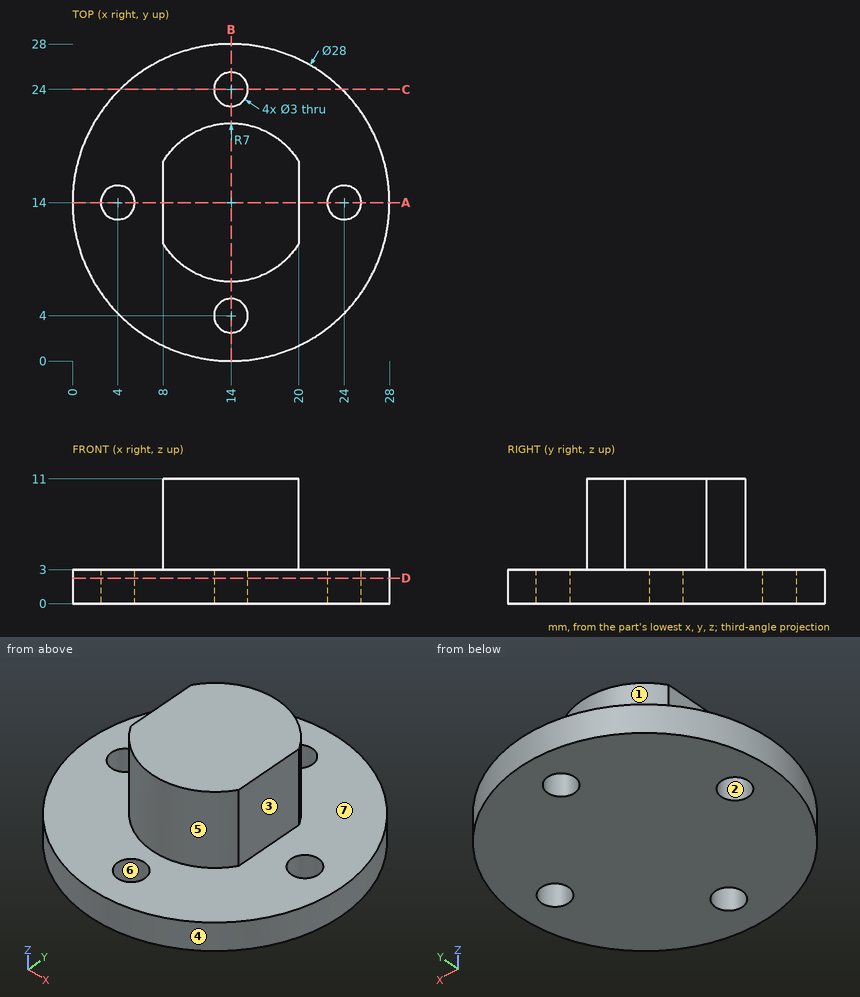
Can you work these out from the drawing? Everything is in mm from the part's minimum corner. A direction names the side the tool comes from. Round coordinates to 2 decimals unless told otherwise and drop trailing zeros. Loops run counter-clockwise (first coordinate to the right, second up) from the corner with the lowest first, then second, coordinate; pieces in that order, holes last. Notation, with made-up numbers: (64.5, -38) - (70.5, -38) arc R27 ccw to (70.5, -10) - close; hole circle Ø6 at (-16, 73.25). An arc over 180 degrees is marked (long way). Answer in a Markdown table with one row per item. Add a question column.
(1) For the marked faces 1, 2 and 3, which set-ups out of +Z, -Z, +X, -X, +Y, -Y let a thin tool reach every point of the face, with its end or its side?
(2) If we section it at C-C (y = 24): Please give me the cut outline in (x, z).
(3) I need wall thicknesses on line 1 along Y through (x, z) = (14, 1.3); line 2 along X through (y, z) = (14.25, 1.5); line 3 along Z through (x, y) = (22.25, 17.25). Which ranges of each line are inside material? Lowest first, please.
(4) If we section it at B-B (x = 14): Please give me the cut outline in (y, z), plus the area to 3 significant figures.
(5) I'm going to push flat-ended pins straight in: pin 1 (4 mm diameter, centred on x = 4, y = 14, fed in from +Z); pin 2 (3 mm diameter, centred on y = 18, z = 9, fed in from -X); pin 3 (1 mm diameter, centred on x = 19, z = 4, fed in from +Y). Where does each tip first touch, or does it pass through?
(6) If we mould it in two halves opening along Y, with no side actions, what happens to the marked faces 4, 5, 6 and 7? For each: pulls with the +Y half, pulls with the -Y half, needs draft (parallel to the pull), parting line crosses it, or undercut.
(7) If we section it at A-A (y = 14): Please give me the cut outline in (x, z), plus the area to 3 significant figures.
(8) If we section it at D-D (z = 2.25): Please give me the cut outline in (x, y).
Model answer:
| question | item | result |
|---|---|---|
| 1 | face 1 | +Z, +Y |
| 1 | face 2 | +Z, -Z |
| 1 | face 3 | +Z, +X, +Y, -Y |
| 2 | outline | (4.2, 0) - (12.5, 0) - (12.5, 3) - (4.2, 3) - close; (15.5, 0) - (23.8, 0) - (23.8, 3) - (15.5, 3) - close |
| 3 | line 1 | y = 0 to 2.5, 5.5 to 22.5, 25.5 to 28 |
| 3 | line 2 | x = 0 to 2.52, 5.48 to 22.52, 25.48 to 28 |
| 3 | line 3 | z = 0 to 3 |
| 4 | outline | (0, 0) - (2.5, 0) - (2.5, 3) - (0, 3) - close; (5.5, 0) - (22.5, 0) - (22.5, 3) - (21, 3) - (21, 11) - (7, 11) - (7, 3) - (5.5, 3) - close; (25.5, 0) - (28, 0) - (28, 3) - (25.5, 3) - close |
| 4 | area | 178 mm² |
| 5 | pin 1 | stops at z = 3 |
| 5 | pin 2 | stops at x = 8 |
| 5 | pin 3 | stops at y = 19.36 |
| 6 | face 4 | parting line crosses it |
| 6 | face 5 | pulls with the -Y half |
| 6 | face 6 | undercut |
| 6 | face 7 | needs draft |
| 7 | outline | (0, 0) - (2.5, 0) - (2.5, 3) - (0, 3) - close; (5.5, 0) - (22.5, 0) - (22.5, 3) - (20, 3) - (20, 11) - (8, 11) - (8, 3) - (5.5, 3) - close; (25.5, 0) - (28, 0) - (28, 3) - (25.5, 3) - close |
| 7 | area | 162 mm² |
| 8 | outline | circle Ø28 at (14, 14); hole circle Ø3 at (4, 14); hole circle Ø3 at (14, 4); hole circle Ø3 at (14, 24); hole circle Ø3 at (24, 14) |
